```python
from build123d import *

# Parameters (mm, degrees)
PAD_DEPTH       = 2.5
SKETCH002_R     = 1.6
POCKET001_DEPTH = 4.001


with BuildPart() as part:
    # Sketch → Pad (new body, symmetric)
    with BuildSketch(Plane.XZ):
        Polygon((-27.15, 0), (27.15, 0), (32.15, 0), (32.15, -4), (-32.15, -4), (-32.15, 0), align=None)
    extrude(amount=PAD_DEPTH, both=True)

    # Sketch002 → Pocket001 (cut, through all)
    with BuildSketch(Plane.XY):
        with Locations((29.65, 0)):
            Circle(SKETCH002_R)
        with Locations((-29.65, 0)):
            Circle(SKETCH002_R)
    extrude(amount=-POCKET001_DEPTH, mode=Mode.SUBTRACT)


solid = part.part
```
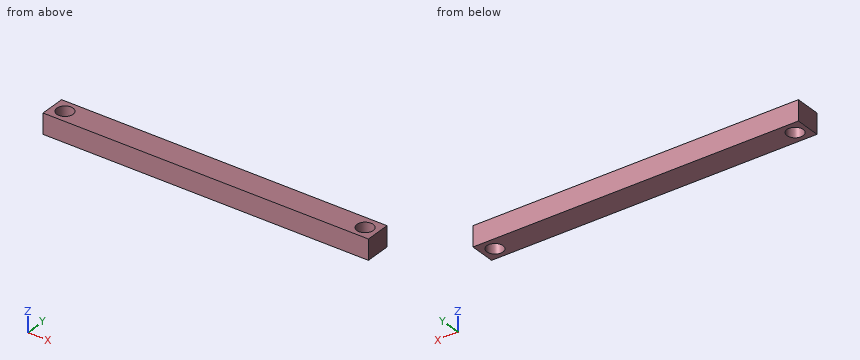
Can you work these out from the model? Positions are in its coordinate system, mm. Give positions to 0.01 mm unless a question says otherwise; leave off trailing zeros. Loops run counter-clockwise (first coordinate to the right, second up) from the corner with the lowest first, then second, coordinate; pieces in that order, holes last. Notation, with made-up numbers: M 14.25,-36 L 65.25,-36 A14 cw 65.25,-25 Z; hole C 44.25,10 d10. An arc over 180 degrees is marked long. Use one line per item in the form item = value. Start each with the question number.
(1) I want a section at C-C, the plane z = -1.4. Write out the boundary of the cut face in (x, y), and give its area (3 significant figures).
(2) Please list where these lines run through material, in increasing order: line 1 (X direction, y = 0.15, z = -2.9); line 2 (Y direction, x = 29.65, z = -2); line 3 (X direction, y = -0.9, z = -3.55).
(3) I want a section at A-A, the plane x = 29.65. Write out the boundary of the cut face in (y, z), and give its area (3 significant figures).
(4) I want a section at B-B, the plane y = 0. Write out the boundary of the cut face in (x, z), and give its area (3 significant figures).
Worked out:
q1.outline = M -32.15,-2.5 L 32.15,-2.5 L 32.15,2.5 L -32.15,2.5 Z; hole C -29.65,0 d3.2; hole C 29.65,0 d3.2
q1.area = 305 mm²
q2.line_1 = -32.15 to -31.24, -28.06 to 28.06, 31.24 to 32.15
q2.line_2 = -2.5 to -1.6, 1.6 to 2.5
q2.line_3 = -32.15 to -30.97, -28.33 to 28.33, 30.97 to 32.15
q3.outline = M -2.5,-4 L -1.6,-4 L -1.6,0 L -2.5,0 Z; M 1.6,-4 L 2.5,-4 L 2.5,0 L 1.6,0 Z
q3.area = 7.20 mm²
q4.outline = M -32.15,-4 L -31.25,-4 L -31.25,0 L -32.15,0 Z; M -28.05,-4 L 28.05,-4 L 28.05,0 L -28.05,0 Z; M 31.25,-4 L 32.15,-4 L 32.15,0 L 31.25,0 Z
q4.area = 232 mm²
